Input: dimensioned drawing with shaded views. Units: mm. Origin: part minimum x, y, z. A direction names the side the tool comes from. Round coordinates to 2 decimals unless told otherwise and drop trailing zeros. Loops run counter-clockwise (first coordinate to the right, second up) from the corner with the lowest first, then second, coordinate; pieces in that order, holes last. Notation, with made-up numbers: (78, 11.25) - (82, 11.25) arc R23 cw to (82, 25.25) - close; hole circle Ø3 at (9, -35). An arc over 180 degrees is marked (long way). Answer as CSV lines item,"result".
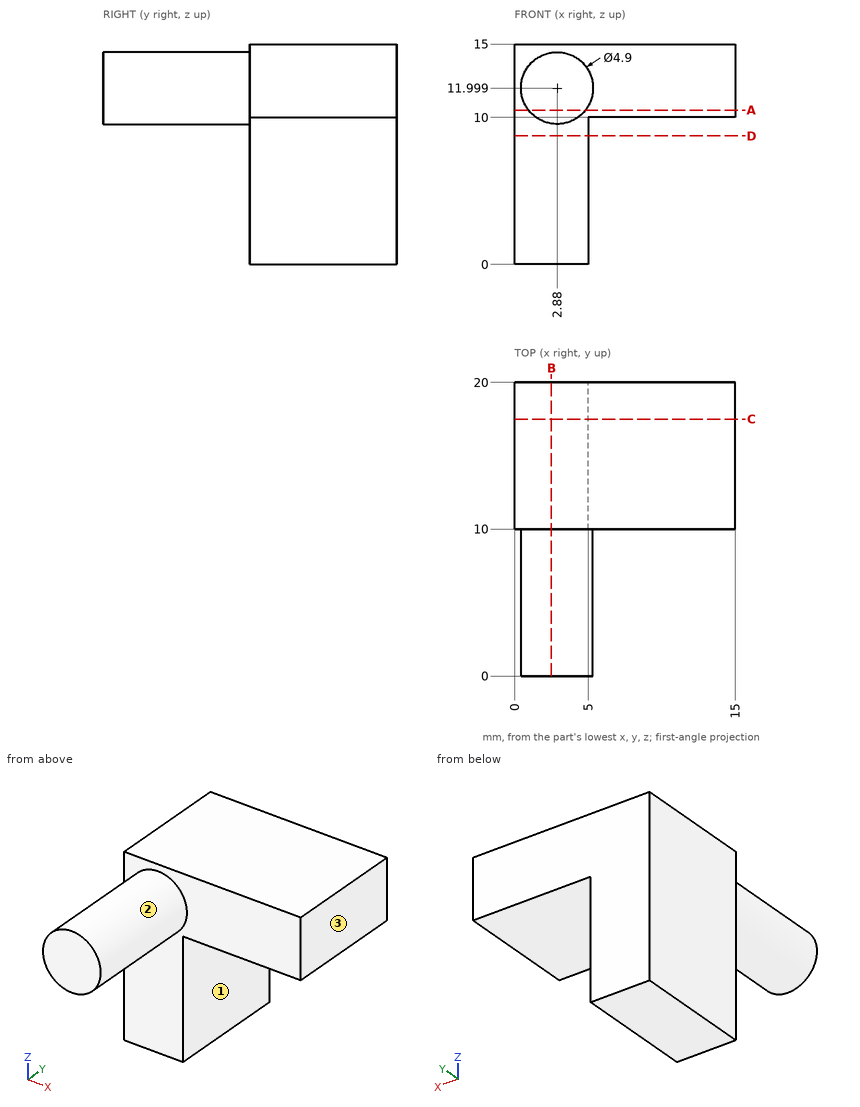
(1) Access query for the marked faces 1, 2 and 3. Directions: +Z, -Z, +X, -X, +Y, -Y. A direction counts if a zero-diameter tool reaches every point of the face in a straight line with its end or side. Return the directions, or none.
Findings below:
face 1,"-Z, +X, +Y, -Y"
face 2,"-Y"
face 3,"+Z, -Z, +X, +Y, -Y"
(2) Section B-B (x = 2.5). Output: boundary loops of the cut face in (y, z), and give its area (3 significant figures).
Findings below:
outline,"(0, 9.58) - (10, 9.58) - (10, 0) - (20, 0) - (20, 15) - (10, 15) - (10, 14.42) - (0, 14.42) - close"
area,"198 mm2"
(3) Pin query (flat end, axial travel): P1, Ø4, axis at x = 13, z = 6.5, coming from the -Y side; P2, Ø3, axis at y = 17.5, z = 4, coming from the -X side; P3, Ø8, axis at x = 7.5, z = 2.5, coming from the -Y side; P4, Ø2, axis at y = 3, z = 12.5, coming from the +X side. Return the tip coordinate at first contact, or that it passes through.
Findings below:
P1,"through"
P2,"x = 0"
P3,"y = 10"
P4,"x = 5.33"
(4) Section A-A (z = 10.5). Output: boundary loops of the cut face in (x, y), and give its area (3 significant figures).
Findings below:
outline,"(0, 10) - (0.94, 10) - (0.94, 0) - (4.82, 0) - (4.82, 10) - (15, 10) - (15, 20) - (0, 20) - close"
area,"189 mm2"
(5) Section C-C (y = 17.5). Output: boundary loops of the cut face in (x, z).
Findings below:
outline,"(0, 0) - (5, 0) - (5, 10) - (15, 10) - (15, 15) - (0, 15) - close"
(6) Section D-D (z = 8.75). Output: boundary loops of the cut face in (x, y).
Findings below:
outline,"(0, 10) - (5, 10) - (5, 20) - (0, 20) - close"
(7) Material intervals for line 1 along Y through (x, z) = (2.75, 1.5); line 2 along X through (y, z) = (18.5, 8); line 3 along Z through (x, y) = (7.75, 15.25), sorted ascending.
Findings below:
line 1,"10 to 20"
line 2,"0 to 5"
line 3,"10 to 15"
